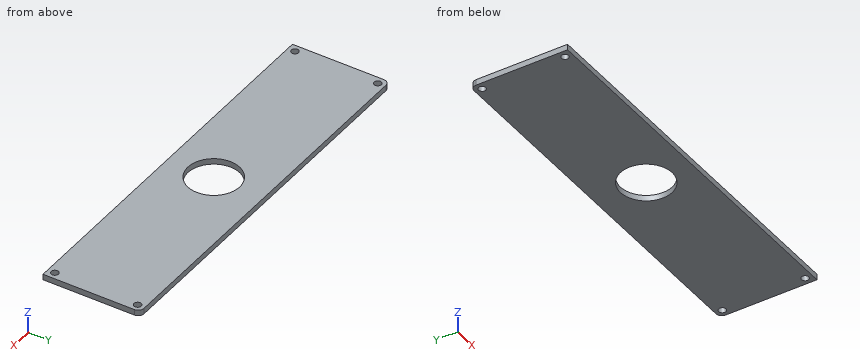
from build123d import *

# Parameters (mm, degrees)
SKETCH_W           = 134
SKETCH_H           = 33.8
PAD_DEPTH          = 2
SKETCH001_R        = 9
POCKET_DEPTH       = 2.001
FILLET_R           = 2
SKETCH002_R        = 1.25
POCKET001_DEPTH    = 278.424154
POLARPATTERN_COUNT = 2


with BuildPart() as part:
    # Sketch → Pad (new body)
    with BuildSketch(Plane.XY):
        Rectangle(SKETCH_W, SKETCH_H)
    extrude(amount=PAD_DEPTH)

    # Sketch001 (on Face6 of Pad) → Pocket (cut, through all)
    with BuildSketch(Plane.XY.offset(2)):
        with Locations((0, -0.9)):
            Circle(SKETCH001_R)
    extrude(amount=-POCKET_DEPTH, mode=Mode.SUBTRACT)

    # Fillet
    fillet_edges = [part.edges().sort_by_distance(p)[0] for p in [
        (-67, 16.9, 1),
        (67, 16.9, 1),
    ]]
    fillet(fillet_edges, radius=FILLET_R)

    # Sketch002 → Pocket001 (cut, through all)
    with BuildSketch(Plane.XY):
        with Locations((-64.5, -14.4)):
            Circle(SKETCH002_R)
    pocket001 = extrude(amount=POCKET001_DEPTH, mode=Mode.SUBTRACT)

    # Mirrored: Pocket001 across YZ
    add(pocket001.mirror(Plane.YZ), mode=Mode.SUBTRACT)

    # Mirrored001: Pocket001 across XZ
    add(pocket001.mirror(Plane.XZ), mode=Mode.SUBTRACT)

    # PolarPattern: Pocket001 ×2 about axis
    polarpattern_axis = Axis((0, 0, 0), (0, 0, 1))
    for i in range(1, POLARPATTERN_COUNT):
        add(pocket001.rotate(polarpattern_axis, i * 360 / POLARPATTERN_COUNT), mode=Mode.SUBTRACT)


solid = part.part
The model under review builds one solid part; all positions refer to its coordinate system, in mm. Round coordinates to 2 decimals unless told otherwise and drop trailing zeros. Order: outer loops, then holes, each group sorted by start corner. A loop starts at its lowest first (then second) coordinate and runs counter-clockwise, first axis right, second up. Notation, with made-up numbers: (33.25, -28) -> (42.25, -28) arc R20 ccw to (42.25, -20) -> close; hole circle Ø11 at (-20.5, 50.5). An arc over 180 degrees is marked (long way). Write item = value, one per line. Start each with the question number.
Item 1: Consider section B-B on x = 0. Write out the cut boundary in (y, z).
Item 2: Consider section A-A on y = -14.4. Write out the cut boundary in (x, z).
Item 3: Consider section C-C on z = 1.6. Write out the cut boundary in (x, y), plus the area to 3 significant figures.
Item 4: Consider section D-D on y = 5.5. Write out the cut boundary in (x, z), plus the area to 3 significant figures.
Item 5: For line 1 along Y through (x, z) = (-64.5, 0.7); line 2 along X through (y, z) = (14.4, 1.5); line 3 along X through (y, z) = (15, 1.3), list the stretches that pass through material, from the lowest coordinate up.
Conclusion:
q1.outline = (-16.9, 0) -> (-9.9, 0) -> (-9.9, 2) -> (-16.9, 2) -> close; (8.1, 0) -> (16.9, 0) -> (16.9, 2) -> (8.1, 2) -> close
q2.outline = (-67, 0) -> (-65.75, 0) -> (-65.75, 2) -> (-67, 2) -> close; (-63.25, 0) -> (63.25, 0) -> (63.25, 2) -> (-63.25, 2) -> close; (65.75, 0) -> (67, 0) -> (67, 2) -> (65.75, 2) -> close
q3.outline = (-67, -16.9) -> (67, -16.9) -> (67, 14.9) arc R2 ccw to (65, 16.9) -> (-65, 16.9) arc R2 ccw to (-67, 14.9) -> close; hole circle Ø2.5 at (-64.5, -14.4); hole circle Ø2.5 at (-64.5, 14.4); hole circle Ø18 at (0, -0.9); hole circle Ø2.5 at (64.5, -14.4); hole circle Ø2.5 at (64.5, 14.4)
q3.area = 4,250 mm2
q4.outline = (-67, 0) -> (-6.33, 0) -> (-6.33, 2) -> (-67, 2) -> close; (6.33, 0) -> (67, 0) -> (67, 2) -> (6.33, 2) -> close
q4.area = 243 mm2
q5.line_1 = -16.9 to -15.65, -13.15 to 13.15, 15.65 to 16.9
q5.line_2 = -67 to -65.75, -63.25 to 63.25, 65.75 to 67
q5.line_3 = -67 to -65.6, -63.4 to 63.4, 65.6 to 67
